Job drawing, mm, ordinate dimensions from the low corner. One solid piece. A direction names the side the tool comes from. Round coordinates to 2 decimals unless told otherwise and drop trailing zeros. Loops run counter-clockwise (first coordinate to the right, second up) from the corner with the lowest first, then second, coordinate; pieces in that order, holes last. Notation, with made-up numbers: M 41,8.25 L 84,8.25 A27 ccw 84,43.25 Z; hole C -5,42 d9. An arc over 180 degrees is marked long. One line per item, written item: value.
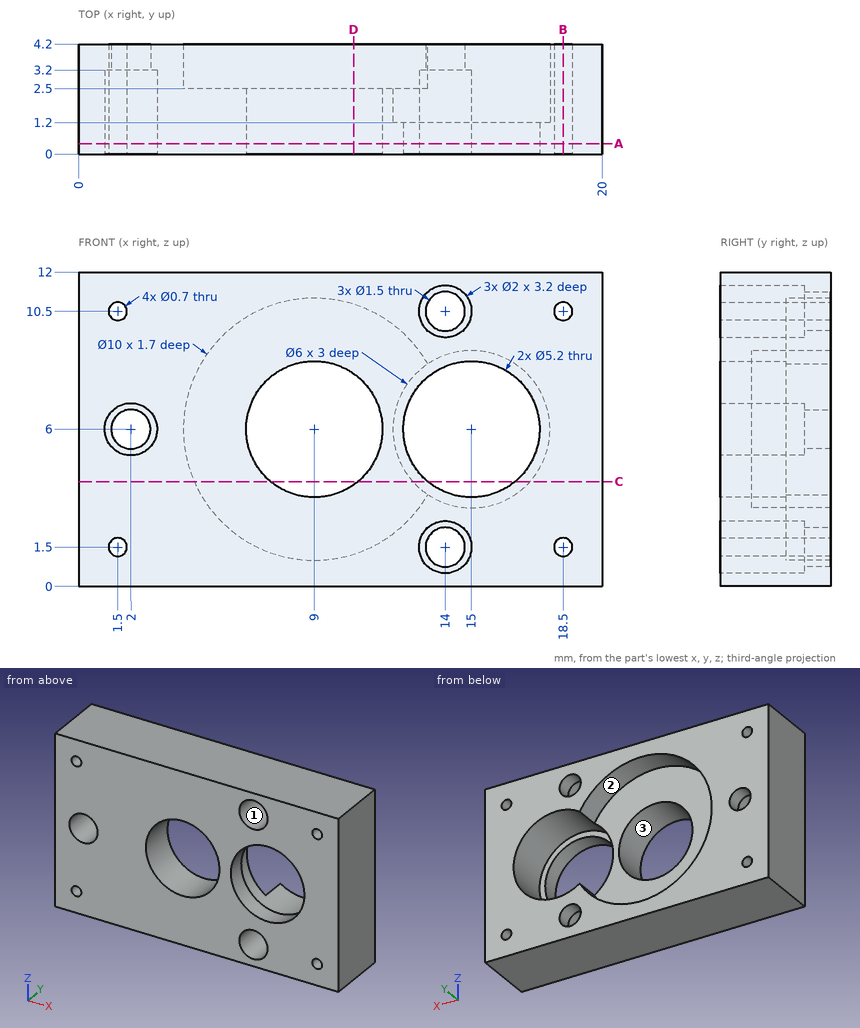
Item 1: Drop flat-ended pins along their axis: P1, Ø1.6, axis at x = 14, z = 1.5, coming from the -Y side; P2, Ø1.2, axis at x = 2, z = 6, coming from the -Y side. Give the stop position or say it passes through.
Check values:
P1: stops at y = 3.2
P2: passes through
Item 2: Wall check: line 1 along X through (y, z) = (1.95, 6); line 2 along X through (y, z) = (0.95, 8.25); line 3 along Z through (x, y) = (13.75, 2.35). Give the ranges that are in metal, low to high.
Check values:
line 1: x = 0 to 1, 3 to 6.4, 11.6 to 12, 18 to 20
line 2: x = 0 to 7.7, 10.3 to 13.7, 16.3 to 20
line 3: z = 0 to 0.53, 2.47 to 3.27, 8.73 to 9.53, 11.47 to 12
Item 3: Slice it at A-A, the plane y = 0.4. Give the number of separate pieces and of enclosed holes in the cut face, and give its area (3 significant figures).
Check values:
separate pieces: 1
enclosed holes: 9
area: 187 mm2
Item 4: Slice it at B-B, the plane x = 18.5. Give the cut face in (y, z).
Check values:
outline: M 0,0 L 4.2,0 L 4.2,1.15 L 0,1.15 Z; M 0,1.85 L 4.2,1.85 L 4.2,10.15 L 0,10.15 Z; M 0,10.85 L 4.2,10.85 L 4.2,12 L 0,12 Z
Item 5: Slice it at C-C, the plane z = 4. Give the cut face in (x, y).
Check values:
outline: M 0,0 L 7.34,0 L 7.34,2.5 L 4.42,2.5 L 4.42,4.2 L 0,4.2 Z; M 10.66,0 L 13.34,0 L 13.34,1.2 L 12.76,1.2 L 12.76,2.5 L 10.66,2.5 Z; M 16.66,0 L 20,0 L 20,4.2 L 17.24,4.2 L 17.24,1.2 L 16.66,1.2 Z
Item 6: Which spindle directions (+Z, -Z, +X, -X, +Y, -Y) get a long thin tool onto all of the face, cutting with end or side? Do the marked faces 1, 2 and 3. Say none if no direction does.
Check values:
face 1: -Y
face 2: +Y
face 3: +Y, -Y
Item 7: Slice it at D-D, the plane x = 10.5. Give the cut face in (y, z), and give its area (3 significant figures).
Check values:
outline: M 0,0 L 4.2,0 L 4.2,1.23 L 2.5,1.23 L 2.5,3.88 L 0,3.88 Z; M 0,8.12 L 2.5,8.12 L 2.5,10.77 L 4.2,10.77 L 4.2,12 L 0,12 Z
area: 23.6 mm2
